Input: part model. Units: mm. Frame: model coordinates. Face numbers are marked on the shaded views. A direction names the side the tool comes from. Coordinates: 2 decimals unless noted, no trailing zeros. Write each loop counter-clockwise with the first axis right and the second up, starting at its lowest first coordinate (ties: lowest second). Pieces come first, ordered by that corner, then holes.
1) Pin query (flat end, axial travel): pin 1 Ø0.9 at (x, z) = (-5, 18) entering from +Y; pin 2 Ø8 at (y, z) = (56, 3) entering from -X; pin 3 Ø6 at (x, y) = (-7, 46) entering from -Z; pin 4 Ø4 at (x, z) = (-8.5, 0.5) entering from -Y. Return the tip coordinate at first contact, or that it passes through.
2) Section query D-D (z = -4). Output: boundary loops of the cut face in (x, y), then the cut area to 3 significant figures.
3) Line query: L1, parallel to Z at x = -2.25, y = -7; L2, parallel to Z at x = -3.95, y = 85; L3, parallel to Y at x = -1.55, z = 5. Output: solid intervals per line, ascending.
4) Section query A-A (y = -7). Output: boundary loops of the cut face in (x, z).
5) Set-up query: the marked faces 1, 2 and 3. Return all of +Z, -Z, +X, -X, +Y, -Y with unobstructed straight access to the full face (end or side cutting, diameter ignored); none if empty.
6) Section query C-C (y = 14.5). Output: boundary loops of the cut face in (x, z).
7) Section query B-B (x = -2.25). State how many separate pieces and enclosed holes the cut face has, then the cut area to 3 significant figures.
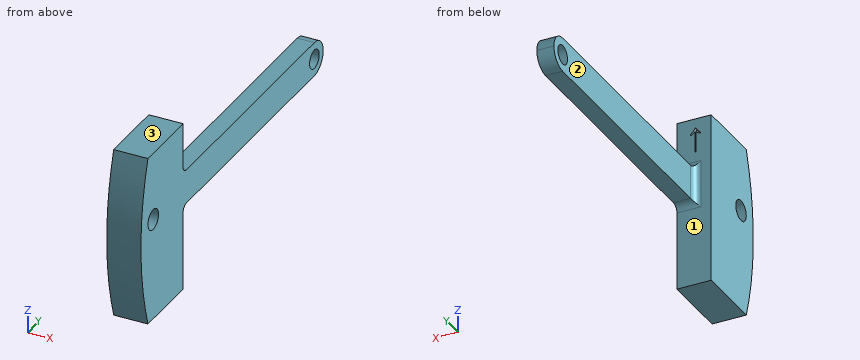
Autodesk Inventor part; units mm, degrees
ref_plane "YZ Plane" through (0, 0, 0) normal (1, 0, 0) x (0, 1, 0)
ref_plane "XZ Plane" through (0, 0, 0) normal (0, 1, 0) x (-1, 0, 0)
ref_plane "XY Plane" through (0, 0, 0) normal (0, 0, 1) x (1, 0, 0)
sketch "スケッチ1" plane through (0, 0, 0) normal (1, 0, 0) x (0, 1, 0)
  line L0 (-10, 25) -> (10, 25)
  line L1 (10, 25) -> (10, -25)
  line L2 (10, -25) -> (-10, -25)
  line L3 (-10, -25) -> (-10, 25)
  line L4 (-10, 25) -> (10, -25) construction
  line L5 (10, 25) -> (-10, -25) construction
  line L6 (10, 0) -> (-14, 0)
  arc A0 (-10, 25) -> (-10, -25) centre (66.125, 0) ccw
  point P0 (0, 0)
  dimension "d0" = 20
  dimension "d1" = 50
  dimension "d9" = 24
extrude "押し出し1" add sketch "スケッチ1" against normal blind 10
sketch "スケッチ2" plane through (0, 0, 0) normal (1, 0, 0) x (0, 0, -1)
  line L0 (-25, 10) -> (25, 10)
  line L1 (-10, 10) -> (0, 10)
  line L2 (0, 10) -> (0, 90)
  line L3 (0, 90) -> (-10, 90)
  line L4 (-10, 90) -> (-10, 10)
  point P0 (0, 0)
  point P1 (0, 10)
  dimension "d4" = 10
  dimension "d5" = 80
  dimension "d6" = 10
extrude "押し出し2" add sketch "スケッチ2" against normal blind 5
sketch "スケッチ3" plane through (0, 0, 0) normal (1, 0, 0) x (0, 0, -1)
  line L0 (25, 10) -> (0, 10)
  point P0 (0, 0)
  point P1 (-5, -7)
  dimension "d12" = 5
  dimension "d13" = 7
hole "穴1" at (0, -7, 5) direction (-1, 0, 0) diameter 6 end through all
sketch "スケッチ4" plane through (0, 0, 0) normal (1, 0, 0) x (0, 0, -1)
  line L0 (0, 90) -> (-10, 90)
  line L1 (0, 10) -> (0, 90)
  point P0 (0, 0)
  point P1 (-5, 85)
  point P2 (-5, 90)
  dimension "d21" = 5
  dimension "d22" = 5
hole "穴2" at (0, 85, 5) direction (-1, 0, 0) diameter 5.5 end through all
fillet "フィレット1" radius 2 3 edges at (-2.5, 10, 0) (-5, 10, 5) (-2.5, 10, 10)
fillet "フィレット2" radius 5 2 edges at (-2.5, 90, 0) (-2.5, 90, 10)
sketch "スケッチ5" plane through (-10, 10, -25) normal (0, 1, 0) x (1, 0, 0)
  line L0 (2.5, -40) -> (7.5, -40) construction
  line L1 (7.5, -40) -> (7.5, -45) construction
  line L2 (7.5, -45) -> (2.5, -45) construction
  line L3 (2.5, -45) -> (2.5, -40) construction
  line L4 (10, -37) -> (10, -50)
  line L5 (10, -50) -> (0, -50)
  line L6 (3.1278, -45.5513) -> (3.1278, -45.2399)
  spline S0 degree 2 poles (3.1278, -45.2399) (3.6122, -45.4821) (3.9978, -45.7293) (4.3933, -46.0407) knots 0 0 0 1 2 2 2
  line L7 (4.3933, -46.0407) -> (4.3933, -40)
  line L8 (4.3933, -40) -> (4.8085, -40)
  line L9 (4.8085, -40) -> (4.8085, -46.0407)
  spline S1 degree 2 poles (4.8085, -46.0407) (5.2485, -45.6156) (6.074, -45.23) knots 0 0 0 1 1 1
  line L10 (6.074, -45.23) -> (6.074, -45.5464)
  spline S2 degree 2 poles (6.074, -45.5464) (5.4808, -46.0753) (4.8728, -46.8365) (4.68, -47.2419) knots 0 0 0 1 2 2 2
  line L11 (4.68, -47.2419) -> (4.4921, -47.2419)
  spline S3 degree 2 poles (4.4921, -47.2419) (4.3389, -46.8909) (3.721, -46.0951) (3.1278, -45.5513) knots 0 0 0 1 2 2 2
  point P0 (10, -25)
  point P1 (7.5, -42.5)
  dimension "d34" = 2.5
  dimension "d35" = 5
  dimension "d36" = 5
  dimension "d37" = 5
extrude "押し出し3" cut sketch "スケッチ5" against normal blind 1
properties part number "受動歩行_ver2"
Answer:
1. pin 1: stops at y = 10
1. pin 2: stops at x = -5
1. pin 3: stops at z = 0
1. pin 4: stops at y = -14
2. outline: (-10, -13.9) - (0, -13.9) - (0, 10) - (-10, 10) - close
2. area: 239 mm2
3. L1: z = -25 to 2, 8 to 25
3. L2: z = 0 to 2.25, 7.75 to 10
3. L3: y = -13.84 to -10, -4 to 82.25, 87.75 to 90
4. outline: (-10, -25) - (0, -25) - (0, 2) - (-10, 2) - close; (-10, 8) - (0, 8) - (0, 25) - (-10, 25) - close
5. face 1: -X, +Y
5. face 2: +Z, -Z, -X, +Y
5. face 3: +Z, +X, -X, +Y, -Y
6. outline: (-5, 0) - (0, 0) - (0, 10) - (-5, 10) - close
7. separate pieces: 1
7. enclosed holes: 2
7. area: 1,870 mm2
